from build123d import *

# Parameters (mm, degrees)
ESQUISSE1_W             = 1.7
ESQUISSE1_H             = 1.2
BOSS_EXTRU_1_DEPTH      = 0.3
BOSS_EXTRU_1_2_DEPTH    = 0.3
BOSS_EXTRU_1_3_DEPTH    = 0.3
BOSS_EXTRU_1_4_DEPTH    = 0.3
ESQUISSE2_W             = 6.2
ESQUISSE2_H             = 6.2
BOSS_EXTRU_2_DEPTH      = 3
ESQUISSE3_W             = 6.2
ESQUISSE3_H             = 6.2
ENL_V_MAT_EXTRU_1_DEPTH = 0.1
ESQUISSE4_R             = 0.6
BOSS_EXTRU_3_DEPTH      = 0.35
ESQUISSE5_R             = 1.675
BOSS_EXTRU_4_DEPTH      = 1.5
CONG_1_R                = 0.1


with BuildPart() as part:
    # Esquisse1 → Boss.-Extru.1 (new body)
    with BuildSketch(Plane(origin=(0, 0, 0), x_dir=(1, 0, 0), z_dir=(0, 1, 0))):
        with Locations((1.05, 5.4)):
            Rectangle(ESQUISSE1_W, ESQUISSE1_H)
    extrude(amount=BOSS_EXTRU_1_DEPTH)



with BuildPart() as body_2:
    # Esquisse1 → Boss.-Extru.1 2 (new body)
    with BuildSketch(Plane(origin=(0, 0, 0), x_dir=(1, 0, 0), z_dir=(0, 1, 0))):
        with Locations((1.05, 0.8)):
            Rectangle(ESQUISSE1_W, ESQUISSE1_H)
    extrude(amount=BOSS_EXTRU_1_2_DEPTH)


with BuildPart() as body_3:
    # Esquisse1 → Boss.-Extru.1 3 (new body)
    with BuildSketch(Plane(origin=(0, 0, 0), x_dir=(1, 0, 0), z_dir=(0, 1, 0))):
        with Locations((5.15, 0.8)):
            Rectangle(ESQUISSE1_W, ESQUISSE1_H)
    extrude(amount=BOSS_EXTRU_1_3_DEPTH)


with BuildPart() as body_4:
    # Esquisse1 → Boss.-Extru.1 4 (new body)
    with BuildSketch(Plane(origin=(0, 0, 0), x_dir=(1, 0, 0), z_dir=(0, 1, 0))):
        with Locations((5.15, 5.4)):
            Rectangle(ESQUISSE1_W, ESQUISSE1_H)
    extrude(amount=BOSS_EXTRU_1_4_DEPTH)


with BuildPart() as part_1:
    add(part.part)

    add(body_2.part)  # Boss.-Extru.2 merges body 2

    add(body_3.part)  # Boss.-Extru.2 merges body 3

    add(body_4.part)  # Boss.-Extru.2 merges body 4
    # Esquisse2 → Boss.-Extru.2 (add)
    with BuildSketch(Plane(origin=(0, 0.3, 0), x_dir=(1, 0, 0), z_dir=(0, 1, 0))):
        with Locations((3.1, 3.1)):
            Rectangle(ESQUISSE2_W, ESQUISSE2_H)
    extrude(amount=BOSS_EXTRU_2_DEPTH)

    # Esquisse3 → Enlèv. mat.-Extru.1 (cut)
    with BuildSketch(Plane(origin=(0, 3.3, 0), x_dir=(1, 0, 0), z_dir=(0, 1, 0))):
        with Locations((3.1, 3.1)):
            Rectangle(ESQUISSE3_W, ESQUISSE3_H)
        with BuildLine():
            Line((0.3, 0.2), (1.8, 0.2))
            ThreePointArc((1.8, 0.2), (1.870710678, 0.229289322), (1.9, 0.3))
            Line((1.9, 0.3), (1.9, 0.35))
            Line((1.9, 0.35), (4.3, 0.35))
            Line((4.3, 0.35), (4.3, 0.3))
            ThreePointArc((4.3, 0.3), (4.329289322, 0.229289322), (4.4, 0.2))
            Line((4.4, 0.2), (5.9, 0.2))
            ThreePointArc((5.9, 0.2), (5.970710678, 0.229289322), (6, 0.3))
            Line((6, 0.3), (6, 1.3))
            ThreePointArc((6, 1.3), (5.970710678, 1.370710678), (5.9, 1.4))
            Line((5.9, 1.4), (5.85, 1.4))
            Line((5.85, 1.4), (5.85, 2.75))
            ThreePointArc((5.85, 2.75), (5.879289322, 2.820710678), (5.95, 2.85))
            Line((5.95, 2.85), (6, 2.85))
            Line((6, 2.85), (6, 3.35))
            Line((6, 3.35), (5.95, 3.35))
            ThreePointArc((5.95, 3.35), (5.879289322, 3.379289322), (5.85, 3.45))
            Line((5.85, 3.45), (5.85, 4.8))
            Line((5.85, 4.8), (5.9, 4.8))
            ThreePointArc((5.9, 4.8), (5.970710678, 4.829289322), (6, 4.9))
            Line((6, 4.9), (6, 5.9))
            ThreePointArc((6, 5.9), (5.970710678, 5.970710678), (5.9, 6))
            Line((5.9, 6), (4.4, 6))
            ThreePointArc((4.4, 6), (4.329289322, 5.970710678), (4.3, 5.9))
            Line((4.3, 5.9), (4.3, 5.85))
            Line((4.3, 5.85), (1.9, 5.85))
            Line((1.9, 5.85), (1.9, 5.9))
            ThreePointArc((1.9, 5.9), (1.870710678, 5.970710678), (1.8, 6))
            Line((1.8, 6), (0.3, 6))
            ThreePointArc((0.3, 6), (0.229289322, 5.970710678), (0.2, 5.9))
            Line((0.2, 5.9), (0.2, 4.9))
            ThreePointArc((0.2, 4.9), (0.229289322, 4.829289322), (0.3, 4.8))
            Line((0.3, 4.8), (0.35, 4.8))
            Line((0.35, 4.8), (0.35, 3.45))
            ThreePointArc((0.35, 3.45), (0.320710678, 3.379289322), (0.25, 3.35))
            Line((0.25, 3.35), (0.2, 3.35))
            Line((0.2, 3.35), (0.2, 2.85))
            Line((0.2, 2.85), (0.25, 2.85))
            ThreePointArc((0.25, 2.85), (0.320710678, 2.820710678), (0.35, 2.75))
            Line((0.35, 2.75), (0.35, 1.4))
            Line((0.35, 1.4), (0.3, 1.4))
            ThreePointArc((0.3, 1.4), (0.229289322, 1.370710678), (0.2, 1.3))
            Line((0.2, 1.3), (0.2, 0.3))
            ThreePointArc((0.2, 0.3), (0.229289322, 0.229289322), (0.3, 0.2))
        make_face(mode=Mode.SUBTRACT)
    extrude(amount=-ENL_V_MAT_EXTRU_1_DEPTH, mode=Mode.SUBTRACT)

    # Esquisse4 → Boss.-Extru.3 (add)
    with BuildSketch(Plane(origin=(0, 3.3, 0), x_dir=(1, 0, 0), z_dir=(0, 1, 0))):
        with Locations((0.9, 5.3)):
            Circle(ESQUISSE4_R)
        with Locations((5.3, 5.3)):
            Circle(ESQUISSE4_R)
        with Locations((0.9, 0.9)):
            Circle(ESQUISSE4_R)
        with Locations((5.3, 0.9)):
            Circle(ESQUISSE4_R)
    extrude(amount=BOSS_EXTRU_3_DEPTH)

    # Esquisse5 → Boss.-Extru.4 (add)
    with BuildSketch(Plane(origin=(0, 3.3, 0), x_dir=(1, 0, 0), z_dir=(0, 1, 0))):
        with Locations((3.1, 3.1)):
            Circle(ESQUISSE5_R)
    extrude(amount=BOSS_EXTRU_4_DEPTH)

    # Congé1
    cong_1_edges = [part_1.edges().sort_by_distance(p)[0] for p in [
        (1.425, 4.8, -3.1),
    ]]
    fillet(cong_1_edges, radius=CONG_1_R)


solid = part_1.part
For this review, take the finished solid that the model builds, in its own axes (mm). A direction names the side the tool comes from. Round coordinates to 2 decimals unless told otherwise and drop trailing zeros. Write each loop counter-clockwise with the first axis right and the second up, starting at its lowest first coordinate (ties: lowest second). Pieces come first, ordered by that corner, then holes. Notation, with made-up numbers: M 24.5,51 L 45.5,51 A18 cw 45.5,76 Z; hole C 66.25,71.5 d5. An arc over 180 degrees is marked long. Write item = value, one per line. Start each with the question number.
(1) We need section B-B (x = 3.1). Give the boundary of the cut face in (y, z) (3 decimals), then the cut area to 3 significant figures.
(2) We need section A-A (z = -3.1). Give the boundary of the cut face in (x, y) (3 decimals).
(3) For line 1 along Z through (x, y) = (5.25, 0.2); line 2 along X through (y, z) = (3.4, -5.25); line 3 along Y through (x, z) = (1.25, -5.25), list the stretches that pass through material, from the lowest coordinate up.
(4) For faces 1 (the face through (5, 0, -5)), 2 (the face through (0.77, 3.473, -4.714)), list the 3-axis set-ups (+Z, -Z, +X, -X, +Y, -Y) from which the entire face can be reached by the end or side of a thin tool; tool diameter is ignored.
(5) Clearance check with a flat-ended pin moving along its axis: pin 1 Ø1.3 at (x, z) = (1, -5) entering from +Y. State where the tip first meets the part, or that it passes through.
(6) We need section D-D (z = -0.9). Give the boundary of the cut face in (x, y), then the cut area to 3 significant figures.
(7) The part is to be moulded in two halves that separate along Z. For faces 3 (the face through (3, 2, 0)), 4 (the face through (0.3, 3.47, -0.93)), 5 (the face through (1, 3.65, -5)), say which applies: +Z half, -Z half, draft (parallel to the pull), parting line (faces both ways), or undercut.
(8) We need section C-C (y = 4.25). Give the boundary of the cut face in (x, z) (3 decimals), then the cut area to 3 significant figures.
Results found:
q1.outline = M 0.3,-6.2 L 3.2,-6.2 L 3.2,-5.85 L 3.3,-5.85 L 3.3,-4.775 L 4.7,-4.775 A0.1 ccw 4.8,-4.675 L 4.8,-1.525 A0.1 ccw 4.7,-1.425 L 3.3,-1.425 L 3.3,-0.35 L 3.2,-0.35 L 3.2,0 L 0.3,0 Z
q1.area = 23.6 mm²
q2.outline = M 0,0.3 L 6.2,0.3 L 6.2,3.2 L 6,3.2 L 6,3.3 L 4.775,3.3 L 4.775,4.7 A0.1 ccw 4.675,4.8 L 1.525,4.8 A0.1 ccw 1.425,4.7 L 1.425,3.3 L 0.2,3.3 L 0.2,3.2 L 0,3.2 Z
q3.line_1 = -6 to -4.8, -1.4 to -0.2
q3.line_2 = 0.3 to 1.5, 4.7 to 5.9
q3.line_3 = 0 to 3.65
q4.face_1 = +Z, -Z, +X, -X, -Y
q4.face_2 = +Y
q5.pin_1 = 3.65
q6.outline = M 0,0.3 L 0.2,0.3 L 0.2,0 L 1.9,0 L 1.9,0.3 L 4.3,0.3 L 4.3,0 L 6,0 L 6,0.3 L 6.2,0.3 L 6.2,3.2 L 6,3.2 L 6,3.3 L 5.9,3.3 L 5.9,3.65 L 4.7,3.65 L 4.7,3.3 L 1.5,3.3 L 1.5,3.65 L 0.3,3.65 L 0.3,3.3 L 0.2,3.3 L 0.2,3.2 L 0,3.2 Z
q6.area = 20.4 mm²
q7.face_3 = +Z half
q7.face_4 = undercut
q7.face_5 = draft
q8.outline = C 3.1,-3.1 d3.35
q8.area = 8.81 mm²
